from build123d import *

# Parameters (mm, degrees)
F0_R     = 18.415
F0_R_2   = 16.51
F1_DEPTH = 25.4
F3_R     = 18.415
F3_R_2   = 16.51
F3_R_3   = 15.4378836309
F4_DEPTH = 2.54
F5_R     = 18.415
F5_R_2   = 16.51
F6_DEPTH = 25.4


with BuildPart() as f1:
    # F0 (on Top) → F1 (new body)
    with BuildSketch(Plane.XY):
        Circle(F0_R)
        Circle(F0_R_2, mode=Mode.SUBTRACT)
    extrude(amount=F1_DEPTH)

    # F3 (on offset) → F4 (join)
    with BuildSketch(Plane.XY.offset(25.4)):
        Circle(F3_R)
        Circle(F3_R_2, mode=Mode.SUBTRACT)
        Circle(F3_R_2)
        Circle(F3_R_3, mode=Mode.SUBTRACT)
    extrude(amount=F4_DEPTH)

    # F5 (on face) → F6 (join)
    with BuildSketch(Plane.XY.offset(27.94)):
        Circle(F5_R)
        Circle(F5_R_2, mode=Mode.SUBTRACT)
    extrude(amount=F6_DEPTH)


solid = f1.part
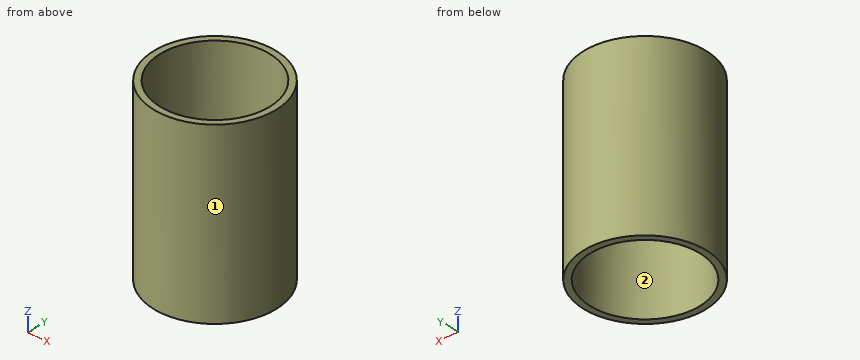
Check sheet for the modelled part. Datum: model origin and axes. Units: mm. Face numbers are marked on the shaded views. Give positions to 0.01 mm unless a question says otherwise; leave off trailing zeros. Loops run counter-clockwise (first coordinate to the right, second up) from the corner with the lowest first, then second, coordinate; pieces in that order, holes last. Notation, with made-up numbers: M 13.25,0 L 67.25,0 A37 cw 67.25,38 Z; hole C 14.5,26.5 d2. An arc over 180 degrees is marked long. Answer as a JSON object with one key per item and string values. Group by question number.
Q1. Material ranges on line 1 along Y through (x, z) = (0, 26.3) (3 decimals); line 2 along Y through (x, z) = (0, 18.75) (3 decimals); line 3 along X through (y, z) = (-7, 26), recorded low to high. Write a range as [from, to].
Q2. Cross-section at A-A on y = 0. Record the cut outline in (x, z) (3 decimals), then the cut area to 3 significant figures.
Q3. Release check for a two-part mould opening along X. For the marked faces 1 and 2 record: released by +X, released by -X, zero draft, split by the parting line, or undercut.
Q4. Cross-section at C-C on z = 39. Record the cut outline in (x, y) (3 decimals).
Q5. Go/stop test with flat-tipped pins: P1, Ø10, axis at y = 4, z = 43, coming from the -X side (3 decimals); P2, Ø5, axis at y = -7, z = 13, coming from the +X side; P3, Ø2, axis at x = -4, z = 37, coming from the +Y side; P4, Ø5, axis at x = -8, z = 29.5, coming from the -Y side. Record where each tip stops, or that it passes through.
Evaluation:
{
 "1": {"line 1": "y = [-18.415, -15.438], [15.438, 18.415]", "line 2": "y = [-18.415, -16.51], [16.51, 18.415]", "line 3": "x = [-17.03, -13.76], [13.76, 17.03]"},
 "2": {"outline": "M -18.415,0 L -16.51,0 L -16.51,25.4 L -15.438,25.4 L -15.438,27.94 L -16.51,27.94 L -16.51,53.34 L -18.415,53.34 Z; M 15.438,25.4 L 16.51,25.4 L 16.51,0 L 18.415,0 L 18.415,53.34 L 16.51,53.34 L 16.51,27.94 L 15.438,27.94 Z", "area": "209 mm2"},
 "3": {"face 1": "split by the parting line", "face 2": "undercut"},
 "4": {"outline": "C 0,0 d36.83; hole C 0,0 d33.02"},
 "5": {"P1": "stops at x = -18.415", "P2": "stops at x = 17.86", "P3": "stops at y = 18.17", "P4": "stops at y = -17.57"}
}
